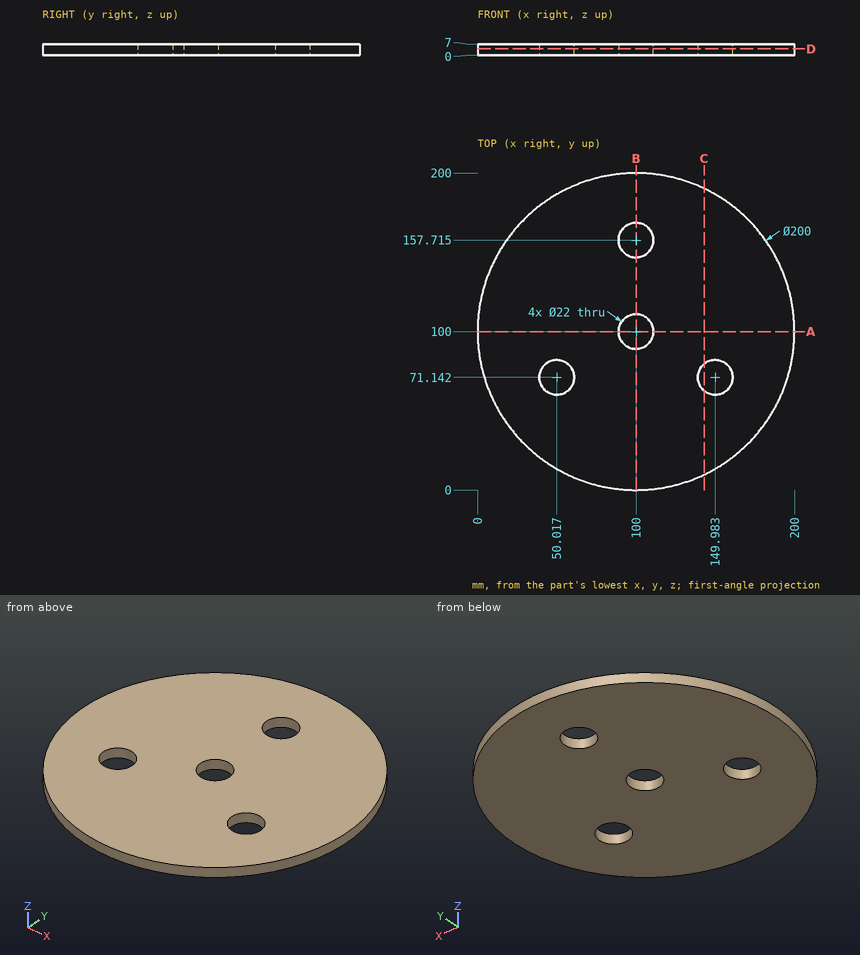
Check sheet for the drawn part. Datum: minimum x, y, z corner. Units: mm. Give positions to 0.01 mm unless a question says otherwise; leave off trailing zeros. Write each loop counter-clockwise with the first axis right and the second up, starting at its lowest first coordinate (ties: lowest second). Pieces come first, ordered by that corner, then holes. Notation, with made-up numbers: M 71.25,18 L 89.25,18 A20 ccw 89.25,37 Z; hole C 4.25,45.25 d11. An arc over 180 degrees is marked long. Write item = value, one per line.
(1) Sectioned sample at D-D (z = 4). Record the cut outline in (x, y) (1 decimal).
Found:
outline = C 100,100 d200; hole C 50,71.1 d22; hole C 100,100 d22; hole C 100,157.7 d22; hole C 150,71.1 d22
(2) Sectioned sample at C-C (x = 143). Record the cut outline in (y, z), then the cut area to 4 significant figures.
Found:
outline = M 9.72,0 L 62.64,0 L 62.64,7 L 9.72,7 Z; M 79.64,0 L 190.28,0 L 190.28,7 L 79.64,7 Z
area = 1,145 mm2
(3) Sectioned sample at A-A (y = 100). Record the cut outline in (x, z).
Found:
outline = M 0,0 L 89,0 L 89,7 L 0,7 Z; M 111,0 L 200,0 L 200,7 L 111,7 Z
(4) Go/stop test with flat-tipped pins: pin 1 Ø2 at (x, z) = (78.5, 4) entering from -Y; pin 2 Ø1 at (y, z) = (31, 4) entering from -X (1 decimal); pin 3 Ø1.5 at (x, z) = (89, 2.5) entering from +Y. Record where each tip stops, or that it passes through.
Found:
pin_1 = 2.12
pin_2 = 27.1
pin_3 = 199.47
(5) Sectioned sample at B-B (x = 100). Record the cut outline in (y, z) (1 decimal), then the cut area to 3 significant figures.
Found:
outline = M 0,0 L 89,0 L 89,7 L 0,7 Z; M 111,0 L 146.7,0 L 146.7,7 L 111,7 Z; M 168.7,0 L 200,0 L 200,7 L 168.7,7 Z
area = 1,090 mm2
(6) Material ranges on line 1 (Y direction, x = 100, z = 2) (1 decimal); line 2 (Y direction, x = 95, z = 3) (1 decimal); line 3 (X direction, y = 62.5, z = 4.5) (1 decimal), recorded low to high.
Found:
line_1 = 0 to 89, 111 to 146.7, 168.7 to 200
line_2 = 0.1 to 90.2, 109.8 to 147.9, 167.5 to 199.9
line_3 = 7.3 to 43.2, 56.8 to 143.2, 156.8 to 192.7
